from build123d import *

# Parameters (mm, degrees)
SKETCH2_R           = 14.5
SKETCH2_R_2         = 12.5
BOSS_EXTRUDE1_DEPTH = 5
BOSS_EXTRUDE2_START = -4
SKETCH2_3_R         = 14.5
BOSS_EXTRUDE2_DEPTH = 4
SKETCH3_R           = 4.1
CUT_EXTRUDE1_DEPTH  = 2


with BuildPart() as part:
    # Sketch2 → Boss-Extrude1 (new body)
    with BuildSketch(Plane(origin=(0, 0, 0), x_dir=(1, 0, 0), z_dir=(0, 1, 0))):
        with Locations(Location((0, 0, 0), (0, 0, 270))):
            Circle(SKETCH2_R)
        with Locations(Location((0, 0, 0), (0, 0, 270))):
            Circle(SKETCH2_R_2, mode=Mode.SUBTRACT)
    extrude(amount=BOSS_EXTRUDE1_DEPTH)

    # Sketch2_3 → Boss-Extrude2 (add)
    with BuildSketch(Plane(origin=(0, 0, 0), x_dir=(1, 0, 0), z_dir=(0, 1, 0)).offset(BOSS_EXTRUDE2_START)):
        with Locations(Location((0, 0, 0), (0, 0, 270))):
            Circle(SKETCH2_3_R)
    extrude(amount=BOSS_EXTRUDE2_DEPTH)

    # Sketch3 → Cut-Extrude1 (cut)
    with BuildSketch(Plane(origin=(0, 0, 0), x_dir=(1, 0, 0), z_dir=(0, 1, 0))):
        with Locations(Location((0, 0, 0), (0, 0, 270))):
            Circle(SKETCH3_R)
    extrude(amount=-CUT_EXTRUDE1_DEPTH, mode=Mode.SUBTRACT)


solid = part.part
Source: CAD feature listing. Evaluate the final solid. Frame: model axes, mm. A direction names the side the tool comes from. Round coordinates to 2 decimals unless told otherwise and drop trailing zeros. Write each loop counter-clockwise with the first axis right and the second up, starting at its lowest first coordinate (ties: lowest second). Pieces come first, ordered by that corner, then holes. Notation, with made-up numbers: M 39,59 L 96,59 A12 ccw 96,66 Z; hole C 9.5,77.5 d4. An arc over 180 degrees is marked long. One line per item, written item: value. Start each with the question number.
Item 1: Section query B-B (y = 4). Return the cut outline in (x, z), plus the area to 3 significant figures.
Item 2: Section query A-A (x = 0). Return the cut outline in (y, z), plus the area to 3 significant figures.
Item 3: Pin query (flat end, axial travel): pin 1 (9.5 mm diameter, centred on x = 0, z = 0, fed in from +Y); pin 2 (1 mm diameter, centred on y = -2.5, z = -2, fed in from -X); pin 3 (4 mm diameter, centred on x = -8, y = 2.5, fed in from +Z). Return the tip coordinate at first contact, or that it passes through.
Item 4: Section query C-C (z = -12). Return the cut outline in (x, y).
Item 5: Set-up query: faces 1 (the cylindrical face through (4.065, -0.986, -0.534)), 2 (the flat face through (0, -4, 0)). Return all of +Z, -Z, +X, -X, +Y, -Y with unobstructed straight access to the full face (end or side cutting, diameter ignored); none if empty.
Item 6: Mould query, pull axis X, two halves, no side actions, for faces 3 (the cylindrical face through (3.755, 2.465, 11.923)), 4 (the flat face through (7, 5, -11)), 5 (the cylindrical face through (-5.554, 0.437, 13.394)). Classes: pulls with the +X half, pulls with the -X half, needs draft (parallel to the pull), parting line crosses it, or undercut.
Item 7: Section query D-D (z = 6.25). Return the cut outline in (x, y), plus the area to 3 significant figures.
Item 8: Ray query, L1, parallel to X at y = 1.1, z = 0; L2, parallel to X at y = -1.5, z = 0; L3, parallel to Z at x = -9.5, y = 1.75. Return the intervals inside material, ascending. Write a range as from..to.
Result set:
1. outline: C 0,0 d29; hole C 0,0 d25
1. area: 170 mm²
2. outline: M -4,-14.5 L 5,-14.5 L 5,-12.5 L 0,-12.5 L 0,-4.1 L -2,-4.1 L -2,4.1 L 0,4.1 L 0,12.5 L 5,12.5 L 5,14.5 L -4,14.5 Z
2. area: 120 mm²
3. pin 1: stops at y = 0
3. pin 2: stops at x = -14.42
3. pin 3: stops at z = 13.2
4. outline: M -8.14,-4 L 8.14,-4 L 8.14,5 L 3.5,5 L 3.5,0 L -3.5,0 L -3.5,5 L -8.14,5 Z
5. face 1: +Y
5. face 2: +Z, -Z, +X, -X, -Y
6. face 3: undercut
6. face 4: needs draft
6. face 5: parting line crosses it
7. outline: M -13.08,-4 L 13.08,-4 L 13.08,5 L 10.83,5 L 10.83,0 L -10.83,0 L -10.83,5 L -13.08,5 Z
7. area: 127 mm²
8. L1: x = -14.5..-12.5, 12.5..14.5
8. L2: x = -14.5..-4.1, 4.1..14.5
8. L3: z = -10.95..-8.12, 8.12..10.95
